The model under review builds one solid part; all positions refer to its coordinate system, in mm. Face numbers are marked on the shaded views. A direction names the side the tool comes from. Coordinates: 2 decimals unless noted, no trailing zeros. Loops run counter-clockwise (first coordinate to the right, second up) from the corner with the lowest first, then second, coordinate; pieces in that order, holes last. Notation, with made-up numbers: M 76.5,42.25 L 133.5,42.25 A17 ccw 133.5,66.25 Z; hole C 68.25,31 d7. An arc over 180 degrees is marked long. Use CSV: the item, a comma, the result in double quotes. Start each with the question number.
from build123d import *

# Parameters (mm, degrees)
SKETCH3_W             = 100
SKETCH3_H             = 100
BOSS_EXTRUDE1_DEPTH   = 3
SKETCH5_W             = 100
SKETCH5_H             = 18
BOSS_EXTRUDE2_DEPTH   = 3
SKETCH6_W             = 100
SKETCH6_H             = 18
BOSS_EXTRUDE3_DEPTH   = 3
SKETCH7_W             = 106
SKETCH7_H             = 18
BOSS_EXTRUDE4_DEPTH   = 3
SKETCH9_W             = 106
SKETCH9_H             = 18
BOSS_EXTRUDE5_DEPTH   = 3
F_8_0MM_DOWEL_HOLE1_D = 8
F_4_0MM_DOWEL_HOLE1_D = 4


with BuildPart() as part:
    # Sketch3 → Boss-Extrude1 (new body)
    with BuildSketch(Plane(origin=(0, 0, 0), x_dir=(1, 0, 0), z_dir=(0, 1, 0))):
        with Locations((50, -50)):
            Rectangle(SKETCH3_W, SKETCH3_H)
    extrude(amount=BOSS_EXTRUDE1_DEPTH)

    # Sketch5 → Boss-Extrude2 (add)
    with BuildSketch(Plane.XY.offset(100)):
        with Locations((50, 9)):
            Rectangle(SKETCH5_W, SKETCH5_H)
    extrude(amount=BOSS_EXTRUDE2_DEPTH)

    # Sketch6 → Boss-Extrude3 (add)
    with BuildSketch(Plane(origin=(0, 0, 0), x_dir=(-1, 0, 0), z_dir=(0, 0, -1))):
        with Locations((-50, 9)):
            Rectangle(SKETCH6_W, SKETCH6_H)
    extrude(amount=BOSS_EXTRUDE3_DEPTH)

    # Sketch7 → Boss-Extrude4 (add)
    with BuildSketch(Plane.ZY):
        with Locations((50, 9)):
            Rectangle(SKETCH7_W, SKETCH7_H)
    extrude(amount=BOSS_EXTRUDE4_DEPTH)

    # Sketch9 → Boss-Extrude5 (add)
    with BuildSketch(Plane(origin=(100, 0, 0), x_dir=(0, 0, -1), z_dir=(1, 0, 0))):
        with Locations((-50, 9)):
            Rectangle(SKETCH9_W, SKETCH9_H)
    extrude(amount=BOSS_EXTRUDE5_DEPTH)

    # Ø8.0mm Dowel Hole1 (through all)
    with Locations(Plane(origin=(0, 3, 0), x_dir=(1, 0, 0), z_dir=(0, 1, 0))):
        with Locations((15, -88)):
            Hole(F_8_0MM_DOWEL_HOLE1_D / 2)

    # Ø4.0mm Dowel Hole1 (through all)
    with Locations(Plane(origin=(0, 3, 0), x_dir=(1, 0, 0), z_dir=(0, 1, 0))):
        with Locations((89, -88)):
            Hole(F_4_0MM_DOWEL_HOLE1_D / 2)


solid = part.part
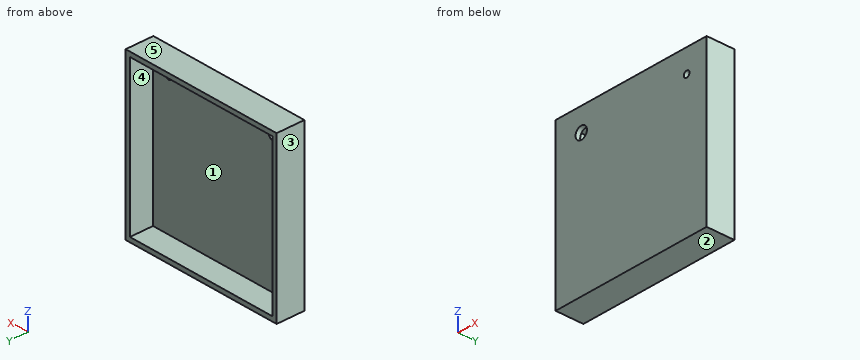
1. To check wall thickness, follow line 1 along X through (y, z) = (0.95, 88); line 2 along X through (y, z) = (3.5, 12); line 3 along Z through (x, y) = (89, 1). State the ranges of each line that lie inside material, in increasing order.
2. Add section A-A (z = 88). Write out the cut boundary in (x, y), plus the area to 3 significant figures.
3. Add section B-B (x = 89). Write out the cut boundary in (y, z), plus the area to 3 significant figures.
4. For the marked faces 4 and 5, list the 3-axis set-ups (+Z, -Z, +X, -X, +Y, -Y) from which the entire face can be reached by the end or side of a thin tool; tool diameter is ignored.
5. Insertion check: pin 1 Ø10 at (x, z) = (23.5, 73) entering from +Y; pin 2 Ø3 at (x, z) = (89, 88) entering from -Y. Each pin has a flat end and moves straight along its axis. Give the tip position at first contact, or say it passes through.
6. Draft analysis for pull direction X (two halves, no side actions). For the marked faces 1, 2 and 3, state which applies: released by +X, released by -X, zero draft, split by the parting line, or undercut.
7. Add section D-D (z = 16). Write out the cut boundary in (x, y), plus the area to 3 significant figures.
8. Add section C-C (y = 7.5). Write out the cut boundary in (x, z).
Solved:
1,line 1,"x = -3 to 11, 19 to 87, 91 to 103"
1,line 2,"x = -3 to 0, 100 to 103"
1,line 3,"z = -3 to 86, 90 to 103"
2,outline,"M -3,0 L 11,0 L 11,3 L 0,3 L 0,18 L -3,18 Z; M 19,0 L 87,0 L 87,3 L 19,3 Z; M 91,0 L 103,0 L 103,18 L 100,18 L 100,3 L 91,3 Z"
2,area,"372 mm^2"
3,outline,"M 0,-3 L 18,-3 L 18,0 L 3,0 L 3,86 L 0,86 Z; M 0,90 L 3,90 L 3,100 L 18,100 L 18,103 L 0,103 Z"
3,area,"396 mm^2"
4,face 4,"+Y"
4,face 5,"+Z, +X, -X, +Y, -Y"
5,pin 1,"stops at y = 3"
5,pin 2,"passes through"
6,face 1,"undercut"
6,face 2,"zero draft"
6,face 3,"released by -X"
7,outline,"M -3,0 L 103,0 L 103,18 L 100,18 L 100,3 L 0,3 L 0,18 L -3,18 Z"
7,area,"408 mm^2"
8,outline,"M -3,-3 L 103,-3 L 103,103 L -3,103 Z; hole M 0,0 L 100,0 L 100,100 L 0,100 Z"
